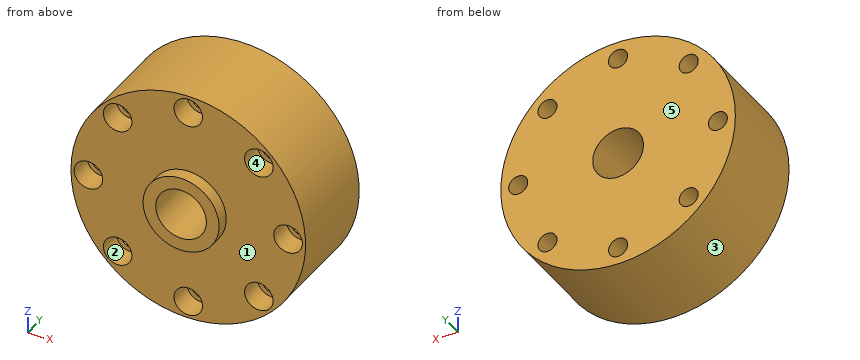
Autodesk Inventor part; units mm, degrees
ref_plane "YZ Plane" through (0, 0, 0) normal (1, 0, 0) x (0, 1, 0)
ref_plane "XZ Plane" through (0, 0, 0) normal (0, 1, 0) x (-1, 0, 0)
ref_plane "XY Plane" through (0, 0, 0) normal (0, 0, 1) x (1, 0, 0)
sketch "Sketch1" plane through (0, 0, 0) normal (0, 1, 0) x (-1, 0, 0)
  circle A0 centre (0, 0) radius 37
  circle A1 centre (0, 0) radius 12
  circle A2 centre (0, 0) radius 8
  circle A3 centre (0, 0) radius 31.5 construction
  circle A4 centre (31.5, 0) radius 3
  circle A5 centre (31.5, 0) radius 4.5
  circle A6 centre (22.2739, 22.2739) radius 3
  circle A7 centre (22.2739, 22.2739) radius 4.5
  circle A8 centre (0, 31.5) radius 3
  circle A9 centre (0, 31.5) radius 4.5
  circle A10 centre (-22.2739, 22.2739) radius 3
  circle A11 centre (-22.2739, 22.2739) radius 4.5
  circle A12 centre (-31.5, 0) radius 3
  circle A13 centre (-31.5, 0) radius 4.5
  circle A14 centre (-22.2739, -22.2739) radius 3
  circle A15 centre (-22.2739, -22.2739) radius 4.5
  circle A16 centre (0, -31.5) radius 3
  circle A17 centre (0, -31.5) radius 4.5
  circle A18 centre (22.2739, -22.2739) radius 3
  circle A19 centre (22.2739, -22.2739) radius 4.5
  dimension "d3" = 63
  dimension "d0" = 74
  dimension "d1" = 24
  dimension "d2" = 16
  dimension "d4" = 6
  dimension "d5" = 9
  dimension "d8" = 360
extrude "Extrusion1" add sketch "Sketch1" along normal blind 30 contours A0 | A1 | A5 | A7 | A9 | A11 | A13 | A15 | A17 | A19
extrude "Extrusion2" cut sketch "Sketch1" along normal blind 7.2 contours A4 | A5 | A6 | A7 | A8 | A9 | A11 | A12 | A13 | A14 | A15 | A16 | A17 | A18 | A19
extrude "Extrusion3" add sketch "Sketch1" against normal blind 4 contours A1
properties part number "LoadCell" material "Stainless Steel"
The listing builds one solid part. Answer for the finished solid, in the listing's coordinates (mm). Face numbers are marked on the shaded views. A direction names the side the tool comes from. Round coordinates to 2 decimals unless told otherwise and drop trailing zeros. Loops run counter-clockwise (first coordinate to the right, second up) from the corner with the lowest first, then second, coordinate; pieces in that order, holes last. Notation, with made-up numbers: (-38.75, -6) - (16.25, -6) arc R15 ccw to (16.25, 10) - close; hole circle Ø11 at (-16, 46). An arc over 180 degrees is marked (long way). Return JSON: item names as keys, results as strings. Group by question number.
1. Consider probe 1 along Z at (x, y) = (0, 5.5); probe 2 along Z at (x, y) = (0, 13); probe 3 along X at (y, z) = (10, 23). Determine where each line is inside the solid, lowest interval first.
2. The part is cut by section C-C on y = 12. State how many separate pieces and enclosed holes the cut face has, then the cut area to 3 significant figures.
3. The mould has two halves that part along Z. Classify the marked faces 1, 2 and 3: pulls with the +Z half, pulls with the -Z half, needs draft (parallel to the pull), parting line crosses it, or undercut.
4. The part is cut by section B-B on x = 0. Determine the outline of the cut face in (y, z).
5. Which of the six approach directions +Z, -Z, +X, -X, +Y, -Y give full straight-line access (tool end or side, diameter ignored) to the marked faces 4 and 5?
6. The part is cut by section A-A on z = 0. Determine the outline of the cut face in (x, y), then the cut area to 3 significant figures.
7. Each of these flat-tipped pins is pushed along its axis until it touches: P1, Ø2.5, axis at x = 32.5, z = -1.5, coming from the -Y side; P2, Ø1.5, axis at x = 27, y = 25, coming from the -Z side; P3, Ø8, axis at x = 1, y = 12.5, coming from the +Z side; P4, Ø14.5, axis at x = -31.5, z = 0, coming from the +Y side. Where does it stop, or does it pass through?
8. The part is cut by section D-D on z = 31.5. Determine the outline of the cut face in (x, y), then the cut area to 3 significant figures.
Resolved:
{
 "1": {"probe 1": "z = -37 to -36, -27 to -8, 8 to 27, 36 to 37", "probe 2": "z = -37 to -34.5, -28.5 to -8, 8 to 28.5, 34.5 to 37", "probe 3": "x = -28.98 to -25.18, -19.36 to 19.36, 25.18 to 28.98"},
 "2": {"separate pieces": "1", "enclosed holes": "9", "area": "3,870 mm²"},
 "3": {"face 1": "needs draft", "face 2": "undercut", "face 3": "parting line crosses it"},
 "4": {"outline": "(-4, -12) - (0, -12) - (0, -27) - (7.2, -27) - (7.2, -28.5) - (30, -28.5) - (30, -8) - (-4, -8) - close; (-4, 8) - (30, 8) - (30, 28.5) - (7.2, 28.5) - (7.2, 27) - (0, 27) - (0, 12) - (-4, 12) - close; (0, -37) - (30, -37) - (30, -34.5) - (7.2, -34.5) - (7.2, -36) - (0, -36) - close; (0, 36) - (7.2, 36) - (7.2, 34.5) - (30, 34.5) - (30, 37) - (0, 37) - close"},
 "5": {"face 4": "-Y", "face 5": "+Z, -Z, +X, -X, +Y"},
 "6": {"outline": "(-37, 0) - (-36, 0) - (-36, 7.2) - (-34.5, 7.2) - (-34.5, 30) - (-37, 30) - close; (-28.5, 7.2) - (-27, 7.2) - (-27, 0) - (-12, 0) - (-12, -4) - (-8, -4) - (-8, 30) - (-28.5, 30) - close; (8, -4) - (12, -4) - (12, 0) - (27, 0) - (27, 7.2) - (28.5, 7.2) - (28.5, 30) - (8, 30) - close; (34.5, 7.2) - (36, 7.2) - (36, 0) - (37, 0) - (37, 30) - (34.5, 30) - close", "area": "1,370 mm²"},
 "7": {"P1": "stops at y = 7.2", "P2": "stops at z = -26.08", "P3": "stops at z = 37", "P4": "stops at y = 30"},
 "8": {"outline": "(-19.41, 0) - (-4.5, 0) - (-4.5, 7.2) - (-3, 7.2) - (-3, 30) - (-19.41, 30) - close; (3, 7.2) - (4.5, 7.2) - (4.5, 0) - (19.41, 0) - (19.41, 30) - (3, 30) - close", "area": "963 mm²"}
}
